Part model, mm, in its own coordinate system. Coordinates: 2 decimals unless noted, no trailing zeros. Order: outer loops, then holes, each group sorted by start corner. A loop starts at its lowest first (then second) coordinate and runs counter-clockwise, first axis right, second up. Notation, with made-up numbers: (31.5, 57) - (43.5, 57) arc R34 ccw to (43.5, 88) - close; hole circle Ø6 at (37.5, 32). An arc over 180 degrees is marked (long way). Use a Markdown table: item, result. Add a question column.
1) Wall check: L1, parallel to Y at x = 339.5, z = 10.5; L2, parallel to Y at x = -331.5, z = 11.75; L3, parallel to X at y = 335.5, z = 12. Give the ranges that are in metal, low to high. Write a range as [from, to].
2) Two-plate mould, pull along X, no slides. Class faces 1 (the face through (-483.76, -370.93, 6.26)), 2 (the face through (306.208, 238.973, 6.261)), 3 (the face through (-9, 9, 0)): +X half, -X half, draft (parallel to the pull), parting line (faces both ways), or undercut.
3) Drop flat-ended pins along their axis: P1, Ø1.5, axis at y = 116.5, z = 2.5, coming from the +X side; P2, Ø3, axis at y = 128.5, z = 11.5, coming from the +X side; P3, Ø3, axis at y = 227.5, z = 3, coming from the -X side. Give the stop position or say it passes through.
4) Saw through at B-B on y = 208. List the corners of the cut face in (x, z), then the cut area to 3 significant figures.
5) Saw through at C-C on y = -514. List the corners of the cut face in (x, z).
6) Saw through at A-A on z = 6.25. List the corners of the cut face in (x, y).
```python
from build123d import *

# Parameters (mm, degrees)
F0_R     = 609.6
F1_DEPTH = 12.7
F3_D     = 127


with BuildPart() as f1:
    # F0 (on Top) → F1 (new body)
    with BuildSketch(Plane.XY):
        Circle(F0_R)
    extrude(amount=F1_DEPTH)

    # F3 (through all)
    with Locations(Plane.XY.offset(12.7)):
        with Locations((335.509866, 295.30862), (335.509866, -295.30862), (-335.509866, -295.30862), (-335.509866, 295.30862)):
            Hole(F3_D / 2)


solid = f1.part
```
Results are:
| question | item | result |
|---|---|---|
| 1 | L1 | [-506.31, -358.68], [-231.93, 231.93], [358.68, 506.31] |
| 1 | L2 | [-511.59, -358.68], [-231.94, 231.94], [358.68, 511.59] |
| 1 | L3 | [-508.97, -384.67], [-286.35, 286.35], [384.67, 508.97] |
| 2 | face 1 | parting line |
| 2 | face 2 | undercut |
| 2 | face 3 | draft |
| 3 | P1 | x = 598.51 |
| 3 | P2 | x = 596.22 |
| 3 | P3 | x = -566.16 |
| 4 | outline | (-573.02, 0) - (573.02, 0) - (573.02, 12.7) - (-573.02, 12.7) - close |
| 4 | area | 14,600 mm2 |
| 5 | outline | (-327.74, 0) - (327.74, 0) - (327.74, 12.7) - (-327.74, 12.7) - close |
| 6 | outline | circle Ø1219.2 at (0, 0); hole circle Ø127 at (-335.51, -295.31); hole circle Ø127 at (-335.51, 295.31); hole circle Ø127 at (335.51, -295.31); hole circle Ø127 at (335.51, 295.31) |
